CAD build for the part. Positions are in the model's coordinates, mm. A direction names the side the tool comes from. Round coordinates to 2 decimals unless told otherwise and drop trailing zeros. Write each loop counter-clockwise with the first axis right and the second up, starting at its lowest first coordinate (ties: lowest second). Pieces come first, ordered by that corner, then holes. Notation, with made-up numbers: (49.25, -33.5) - (66.25, -33.5) arc R29 ccw to (66.25, -5.5) - close; hole circle Ø6 at (-37, -1.5). An arc over 180 degrees is marked (long way). Put each result on its own line as item: value. Start each with the question number.
Item 1: 3-axis set-ups, long thin cutter, end or side, ignore diameter. For faces 1 (the cylindrical face through (11.6, 32.14, -1.52)), 2 (the flat face through (-9.5, 0, 6)): which of +Z, -Z, +X, -X, +Y, -Y reach the whole face in a straight line?
Item 2: Cut at B-B (x = 0). Give the cut face in (y, z) (3 decimals).
Item 3: Cut at D-D (z = 17.75). Give the cut face in (x, y), and give its area (3 significant figures).
Item 4: Mould opens along Z. For faces 3 (the flat face through (12.5, 0, -1)), 4 (the cylindrical face through (-11.3, 0.1, 8.5)), 5 (the flat face through (2, 0, 0)) say: released by +Z, released by -Z, zero draft, split by the parting line, or undercut.
Item 5: Cut at C-C (y = 20). Give the cut face in (x, z) (3 decimals), and give its area (3 significant figures).
Item 6: Drill centre lines: line 1 (Y direction, x = 0, z = -1.95); line 2 (Y direction, x = -11.3, z = 11); line 3 (X direction, y = -4, z = 9.75). Where is each one in solid material? Low to high. Write a range as from..to.
Item 7: Cut at A-A (y = 0). Give the cut face in (x, z) (3 decimals).
Item 8: Pin check, flat tips, straight feed: pin 1 Ø5 at (x, y) = (-8, -23) entering from +Z; pin 2 Ø8 at (x, y) = (7.5, -2) entering from +Z; pin 3 Ø10 at (x, z) = (3.5, 5.5) entering from -Y; pin 4 Ø4 at (y, z) = (-15.5, 7) entering from +X. Stop position of each tip, or through.
```python
from build123d import *

# Parameters (mm, degrees)
SKETCH_1_W                       = 25
SKETCH_1_H                       = 66
SM_BASE_FLANGE_1_DEPTH           = 3
SM_EDGE_FLANGE_1_STRIP_W         = 13.4732
SM_EDGE_FLANGE_1_STRIP_H         = 3
SM_EDGE_FLANGE_1_STRIP_CUT_DEPTH = 66
SM_EDGE_FLANGE_1_DEPTH           = 66
OTHER_START                      = -12.5
OTHER_1_DEPTH                    = 3
OTHER_START_2                    = -3
OTHER_1_2_DEPTH                  = 3
HOLE_WIZARD_M8_2_D               = 9
HOLE_WIZARD_M8_2_DEPTH           = 24.5
HOLE_WIZARD_M8_2_CSINK_D         = 9.05
HOLE_WIZARD_M8_2_CSINK_ANGLE     = 90
HOLE_WIZARD_M8_2_TIP             = 2.703872786
HOLE_WIZARD_M6_1_D               = 5
HOLE_WIZARD_M6_1_DEPTH           = 15
HOLE_WIZARD_M6_1_CSINK_D         = 6.05
HOLE_WIZARD_M6_1_CSINK_ANGLE     = 90
HOLE_WIZARD_M6_1_TIP             = 1.502151548


# Read off the part's stored shape, not the designer's step: 断开-边角1
# Sheet-metal steps are written as plain solids
with BuildPart() as part:
    # Sketch 1 → 基体-法兰1 (new body)
    with BuildSketch(Plane.XY):
        Rectangle(SKETCH_1_W, SKETCH_1_H)
    extrude(amount=-SM_BASE_FLANGE_1_DEPTH)

    # 边线-法兰1 strip (across the edge) → 边线-法兰1 strip cut (cut)
    with BuildSketch(Plane(origin=(-12.5, 33, 0), x_dir=(1, 0, 0), z_dir=(0, -1, 0))):
        with Locations((-3, -1.5)):
            Rectangle(SM_EDGE_FLANGE_1_STRIP_W, SM_EDGE_FLANGE_1_STRIP_H)
    extrude(amount=SM_EDGE_FLANGE_1_STRIP_CUT_DEPTH, mode=Mode.SUBTRACT)

    # 边线-法兰1 section (across the edge) → 边线-法兰1 (add)
    with BuildSketch(Plane(origin=(-12.5, 33, 0), x_dir=(1, 0, 0), z_dir=(0, -1, 0))):
        with BuildLine():
            Line((0, 0.7366), (0, 19))
            Line((0, 19), (3, 19))
            Line((3, 19), (3, 0.7366))
            ThreePointArc((3, 0.7366), (3.215745145, 0.215745145), (3.7366, 0))
            Line((3.7366, 0), (3.7366, -3))
            ThreePointArc((3.7366, -3), (1.094424801, -1.905575199), (0, 0.7366))
        make_face()
    extrude(amount=SM_EDGE_FLANGE_1_DEPTH)

    # Other 1 outline → Other 1 (cut)
    with BuildSketch(Plane.YZ.offset(OTHER_START)):
        with BuildLine():
            ThreePointArc((-33, 16), (-32.121320344, 18.121320344), (-30, 19))
            Line((-30, 19), (-33, 19))
            Line((-33, 19), (-33, 16))
        make_face()
        with BuildLine():
            ThreePointArc((30, 19), (32.121320344, 18.121320344), (33, 16))
            Line((33, 16), (33, 19))
            Line((33, 19), (30, 19))
        make_face()
    extrude(amount=OTHER_1_DEPTH, mode=Mode.SUBTRACT)

    # Other 1 2 outline → Other 1 2 (cut)
    with BuildSketch(Plane.XY.offset(OTHER_START_2)):
        with BuildLine():
            ThreePointArc((9.5, 33), (11.621320344, 32.121320344), (12.5, 30))
            Line((12.5, 30), (12.5, 33))
            Line((12.5, 33), (9.5, 33))
        make_face()
        with BuildLine():
            ThreePointArc((12.5, -30), (11.621320344, -32.121320344), (9.5, -33))
            Line((9.5, -33), (12.5, -33))
            Line((12.5, -33), (12.5, -30))
        make_face()
    extrude(amount=OTHER_1_2_DEPTH, mode=Mode.SUBTRACT)

    # M8 间隙孔2
    with Locations(Plane.XY):
        with Locations((0, 20), (0, -20)):
            CounterSinkHole(HOLE_WIZARD_M8_2_D / 2, HOLE_WIZARD_M8_2_CSINK_D / 2, depth=HOLE_WIZARD_M8_2_DEPTH, counter_sink_angle=HOLE_WIZARD_M8_2_CSINK_ANGLE)
            with Locations((0, 0, -(HOLE_WIZARD_M8_2_DEPTH + HOLE_WIZARD_M8_2_TIP / 2))):  # 118° drill point
                Cone(0, HOLE_WIZARD_M8_2_D / 2, HOLE_WIZARD_M8_2_TIP, mode=Mode.SUBTRACT)

    # M6 螺纹孔1
    with Locations(Plane(origin=(-9.5, 0, 0), x_dir=(0, 0, -1), z_dir=(1, 0, 0))):
        with Locations((-11, 0)):
            CounterSinkHole(HOLE_WIZARD_M6_1_D / 2, HOLE_WIZARD_M6_1_CSINK_D / 2, depth=HOLE_WIZARD_M6_1_DEPTH, counter_sink_angle=HOLE_WIZARD_M6_1_CSINK_ANGLE)
            with Locations((0, 0, -(HOLE_WIZARD_M6_1_DEPTH + HOLE_WIZARD_M6_1_TIP / 2))):  # 118° drill point
                Cone(0, HOLE_WIZARD_M6_1_D / 2, HOLE_WIZARD_M6_1_TIP, mode=Mode.SUBTRACT)


solid = part.part
```
Output values:
1. face 1: +Z, -Z, +X, +Y
1. face 2: +Z, +X, +Y, -Y
2. outline: (-33, -3) - (-24.5, -3) - (-24.5, -0.025) - (-24.525, 0) - (-33, 0) - close; (-15.5, -3) - (15.5, -3) - (15.5, -0.025) - (15.475, 0) - (-15.475, 0) - (-15.5, -0.025) - close; (24.5, -3) - (33, -3) - (33, 0) - (24.525, 0) - (24.5, -0.025) - close
3. outline: (-12.5, -32.44) - (-9.5, -32.44) - (-9.5, 32.44) - (-12.5, 32.44) - close
3. area: 195 mm2
4. face 3: zero draft
4. face 4: undercut
4. face 5: released by +Z
5. outline: (-12.5, 0.737) arc R3.737 ccw to (-8.763, -3) - (-4.5, -3) - (-4.5, -0.025) - (-4.525, 0) - (-8.763, 0) arc R0.737 cw to (-9.5, 0.737) - (-9.5, 19) - (-12.5, 19) - close; (4.5, -3) - (12.5, -3) - (12.5, 0) - (4.525, 0) - (4.5, -0.025) - close
5. area: 102 mm2
6. line 1: -33..-24.5, -15.5..15.5, 24.5..33
6. line 2: -33..-2.5, 2.5..33
6. line 3: -12.5..-9.5
7. outline: (-12.5, 0.737) arc R3.737 ccw to (-8.763, -3) - (12.5, -3) - (12.5, 0) - (-8.763, 0) arc R0.737 cw to (-9.5, 0.737) - (-9.5, 7.975) - (-10.025, 8.5) - (-12.5, 8.5) - close; (-12.5, 13.5) - (-10.025, 13.5) - (-9.5, 14.025) - (-9.5, 19) - (-12.5, 19) - close
8. pin 1: z = 19
8. pin 2: z = 0
8. pin 3: through
8. pin 4: x = -9.5
